Print and shaded views of the part. All mm, measured from the part's lowest x, y and z. A direction names the side the tool comes from. Round coordinates to 2 decimals unless told otherwise and drop trailing zeros. Loops run counter-clockwise (first coordinate to the right, second up) from the corner with the lowest first, then second, coordinate; pieces in that order, holes last. Notation, with made-up numbers: M -11,44 L -2,44 A28 ccw -2,67 Z; hole C 15.5,38.25 d8. An arc over 180 degrees is marked long. One line per item, written item: value. Start each with the question number.
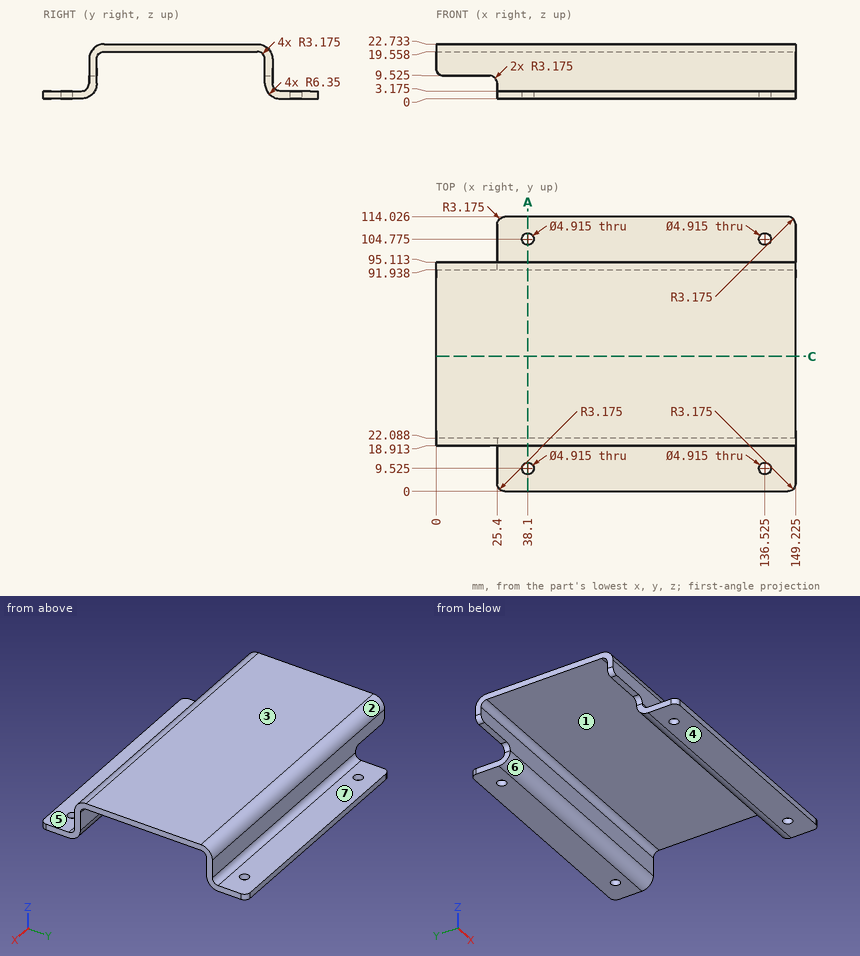
(1) Probe L1, parallel to Y at x = 133.5, z = 10; L2, parallel to Y at x = 38.1, z = 0.8 (1 decimal); L3, parallel to Z at x = 40.5, y = 33.5. List the from-to ranges inside material, lowest first.
(2) Slice it at A-A, the plane x = 38.1. Count the separate pieces of the cut face and the enclosed holes in it, and give its area (3 significant figures).
(3) Mould opens along Y. For the marked faces 1, 2 and 3 say: pulls with the +Y half, pulls with the -Y half, needs draft (parallel to the pull), parting line crosses it, or undercut.
(4) Flat gauge pins, fed straight in: P1, Ø4, axis at x = 136.525, y = 9.525, coming from the +Z side; P2, Ø5, axis at x = 84, z = 9.5, coming from the +Y side; P3, Ø8, axis at x = 136.525, y = 104.775, coming from the +Z side (3 decimals); P4, Ø12, axis at y = 42.5, z = 14.5, coming from the +X side (3 decimals). Where does each tip first touch, or does it go through?
(5) Slice it at C-C, the plane y = 56. List the corners of the cut face in (x, z) (1 decimal), and give its area (3 significant figures).
(6) Which spindle directions (+Z, -Z, +X, -X, +Y, -Y) get a long thin tool onto all of the face, cutting with end or side? Do the marked faces 4, 5, 6 and 7. Say none if no direction does.
Check result:
1. L1: y = 18.91 to 22.09, 91.94 to 95.11
1. L2: y = 0 to 7.1, 12 to 18.8, 95.2 to 102.3, 107.2 to 114
1. L3: z = 19.56 to 22.73
2. separate pieces: 3
2. enclosed holes: 0
2. area: 429 mm^2
3. face 1: undercut
3. face 2: pulls with the +Y half
3. face 3: needs draft
4. P1: passes through
4. P2: stops at y = 95.11
4. P3: stops at z = 3.175
4. P4: stops at x = 149.225
5. outline: M 0,19.6 L 149.2,19.6 L 149.2,22.7 L 0,22.7 Z
5. area: 474 mm^2
6. face 4: -Z, +X, -X, +Y, -Y
6. face 5: +Z, +X, -X, -Y
6. face 6: -Z, +X, -X
6. face 7: +Z, +X, -X, +Y
